Source: CAD feature listing. Evaluate the final solid. Frame: model axes, mm. Give positions to 0.01 mm unless a question says otherwise; leave off trailing zeros. Order: outer loops, then holes, each group sorted by start corner. A loop starts at its lowest first (then second) coordinate and runs counter-clockwise, first axis right, second up. Notation, with made-up numbers: M 56,47 L 72,47 A29 cw 72,76 Z; hole C 76.25,-19.75 d9. An arc over 180 degrees is marked long. Use CSV: the item, a comma, the result in double quotes. Start each with the question number.
1. Pin query (flat end, axial travel): P1, Ø8, axis at y = 4.38, z = 30.74, coming from the +X side. Return the tip coordinate at first contact, or that it passes through.
2. Section query B-B, the plane z = -41.5. Return the cut outline in (x, y), plus the area to 3 significant figures.
3. Section query A-A, the plane y = 3.25. Return the cut outline in (x, z).
4. Section query D-D, the plane y = 7. Return the cut outline in (x, z), plus the area to 3 significant figures.
5. Line query: line 1 along Z through (x, y) = (3, 4.5); line 2 along Z through (x, y) = (3.25, 0.75); line 3 along Y through (x, z) = (6.5, -40). Output: solid intervals per line, ascending. Write a range as [from, to].
6. Section query C-C, the plane x = 8.25. Return the cut outline in (y, z).
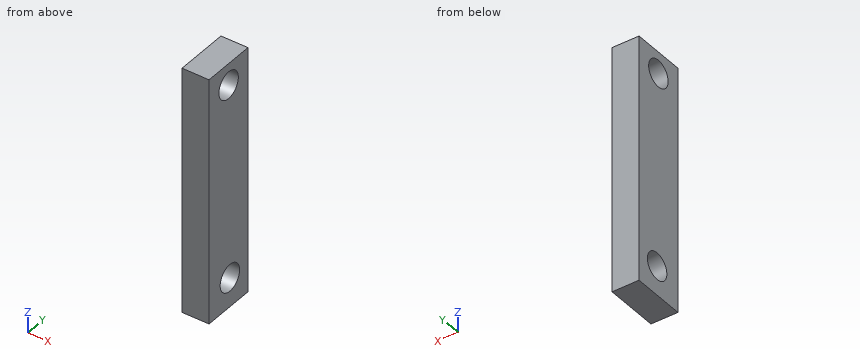
Autodesk Inventor part; units mm, degrees
ref_plane "YZ Plane" through (0, 0, 0) normal (1, 0, 0) x (0, 1, 0)
ref_plane "XZ Plane" through (0, 0, 0) normal (0, 1, 0) x (-1, 0, 0)
ref_plane "XY Plane" through (0, 0, 0) normal (0, 0, 1) x (1, 0, 0)
sketch "Sketch1" plane through (0, 0, 0) normal (1, 0, 0) x (0, 1, 0)
  line L0 (14.3117, 38.8012) -> (-5.6883, 38.8012)
  line L1 (-5.6883, 38.8012) -> (-5.6883, -52.6055)
  line L2 (-5.6883, -52.6055) -> (14.3117, -52.6055)
  line L3 (14.3117, -52.6055) -> (14.3117, 38.8012)
  point P0 (0, 0)
  dimension "d1" = 20
extrude "Extrusion1" add sketch "Sketch1" along normal blind 10
sketch "Sketch2" plane through (0, 0, 0) normal (-1, 0, 0) x (0, 0, 1)
  point P0 (0, 0)
  point P1 (30.7387, 4.3762)
hole "Hole1" at (0, 4.3762, 30.7387) direction (1, 0, 0) diameter 10 end through all
sketch "Sketch3" plane through (0, 0, 0) normal (-1, 0, 0) x (0, 0, 1)
  point P0 (0, 0)
  point P1 (-41.7535, 5.0249)
hole "Hole2" at (0, 5.0249, -41.7535) direction (1, 0, 0) diameter 10 end through all
properties part number "expo arm" material "PVC, Unplasticized"
Result set:
1,P1,"through"
2,outline,"M 0,-5.69 L 10,-5.69 L 10,0.03 L 0,0.03 Z; M 0,10.02 L 10,10.02 L 10,14.31 L 0,14.31 Z"
2,area,"100 mm2"
3,outline,"M 0,-52.61 L 10,-52.61 L 10,-46.43 L 0,-46.43 Z; M 0,-37.08 L 10,-37.08 L 10,25.87 L 0,25.87 Z; M 0,35.61 L 10,35.61 L 10,38.8 L 0,38.8 Z"
4,outline,"M 0,-52.61 L 10,-52.61 L 10,-46.35 L 0,-46.35 Z; M 0,-37.16 L 10,-37.16 L 10,26.48 L 0,26.48 Z; M 0,34.99 L 10,34.99 L 10,38.8 L 0,38.8 Z"
4,area,"737 mm2"
5,line 1,"[-52.61, -46.73], [-36.78, 25.74], [35.74, 38.8]"
5,line 2,"[-52.61, -44.35], [-39.16, 27.3], [34.18, 38.8]"
5,line 3,"[-5.69, 0.34], [9.71, 14.31]"
6,outline,"M -5.69,-52.61 L 14.31,-52.61 L 14.31,38.8 L -5.69,38.8 Z; hole C 4.38,30.74 d10; hole C 5.02,-41.75 d10"
